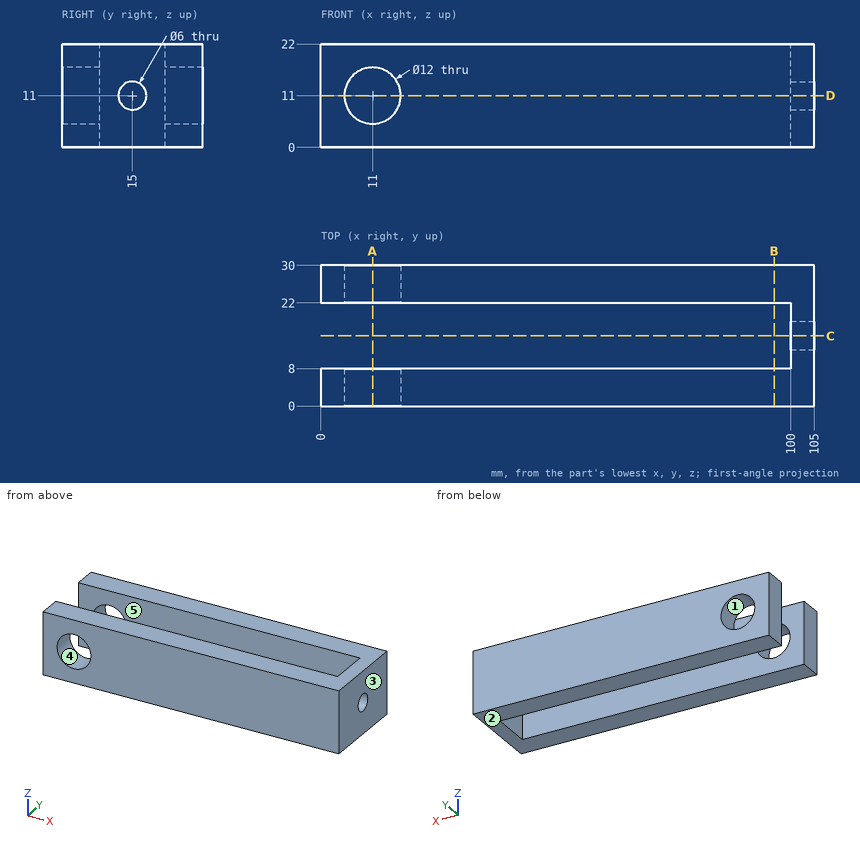
Could you check a few things on this drawing? It's one solid part, dimensions in mm from its lowest x, y, z. A direction names the side the tool comes from. Round coordinates to 2 decimals unless told otherwise and drop trailing zeros. Write each loop counter-clockwise with the first axis right and the second up, starting at its lowest first coordinate (ties: lowest second). Pieces come first, ordered by that corner, then holes. Notation, with made-up numbers: M -38,42 L 9,42 A26 cw 9,77 Z; hole C -7,61.25 d10. An arc over 180 degrees is marked long. Answer as CSV lines item,"result". Start each with the question number.
1. Suppose I cut it at B-B on x = 96.5. Write out the boundary of the cut face in (y, z), then the cut area to 3 significant figures.
2. Suppose I cut it at D-D on z = 11. Write out the boundary of the cut face in (x, y), then the cut area to 3 significant figures.
3. Suppose I cut it at C-C on y = 15. Write out the boundary of the cut face in (x, z).
4. Suppose I cut it at A-A on x = 11. Write out the boundary of the cut face in (y, z), then the cut area to 3 significant figures.
5. I'm going to push a flat-ended pin straight in: pin 1 Ø9.5 at (y, z) = (15, 11) entering from -X. Where does the tip first touch, or does it pass through?
6. I need wall thicknesses on probe 1 along Y at (x, z) = (47.5, 7.5); probe 2 along X at (y, z) = (24.5, 11); probe 3 along X at (y, z) = (11, 10.75). Which ranges of each line are inside material? Lowest first, please.
7. Thinking about a two-plate mould opening in X: for the marked faces 1, 2 and 3, which applies, released by +X, released by -X, zero draft, split by the parting line, or undercut?
8. On a 3-axis mill with a long thin cutter (end or side, diameter ignored), from which of +Z, -Z, +X, -X, +Y, -Y can I reach the whole of each face in a straight line? I mean the marked faces 4 and 5. Say none if no direction works.
Check result:
1,outline,"M 0,0 L 8,0 L 8,22 L 0,22 Z; M 22,0 L 30,0 L 30,22 L 22,22 Z"
1,area,"352 mm2"
2,outline,"M 0,0 L 5,0 L 5,8 L 0,8 Z; M 0,22 L 5,22 L 5,30 L 0,30 Z; M 17,0 L 105,0 L 105,12 L 100,12 L 100,8 L 17,8 Z; M 17,22 L 100,22 L 100,18 L 105,18 L 105,30 L 17,30 Z"
2,area,"1,530 mm2"
3,outline,"M 100,0 L 105,0 L 105,8 L 100,8 Z; M 100,14 L 105,14 L 105,22 L 100,22 Z"
4,outline,"M 0,0 L 8,0 L 8,5 L 0,5 Z; M 0,17 L 8,17 L 8,22 L 0,22 Z; M 22,0 L 30,0 L 30,5 L 22,5 Z; M 22,17 L 30,17 L 30,22 L 22,22 Z"
4,area,"160 mm2"
5,pin 1,"stops at x = 100"
6,probe 1,"y = 0 to 8, 22 to 30"
6,probe 2,"x = 0 to 5, 17 to 105"
6,probe 3,"x = 100 to 105"
7,face 1,"undercut"
7,face 2,"zero draft"
7,face 3,"released by +X"
8,face 4,"+Y, -Y"
8,face 5,"+Z, -Z, -X"
